from build123d import *

# Parameters (mm, degrees)
SKETCH1_W               = 984.25
SKETCH1_H               = 914.4
BOSS_EXTRUDE1_DEPTH     = 11.90625
CUT_EXTRUDE1_DEPTH      = 1
CUT_EXTRUDE1_DEPTH_BACK = 12.90625


with BuildPart() as part:
    # Sketch1 → Boss-Extrude1 (new body)
    with BuildSketch(Plane.XY):
        Rectangle(SKETCH1_W, SKETCH1_H)
    extrude(amount=BOSS_EXTRUDE1_DEPTH)

    # Sketch3 → Cut-Extrude1 (cut, two sides)
    with BuildSketch(Plane.XY.offset(11.90625)) as cut_extrude1_sk:
        Polygon((0, -406.4), (215.9, -406.4), (215.9, -215.9), (-215.9, -215.9), (-215.9, -406.4), align=None)
    extrude(amount=CUT_EXTRUDE1_DEPTH, mode=Mode.SUBTRACT)
    extrude(cut_extrude1_sk.sketch, amount=-CUT_EXTRUDE1_DEPTH_BACK, mode=Mode.SUBTRACT)


solid = part.part
Can you work these out from the model? Positions are in its coordinate system, mm. Coordinates: 2 decimals unless noted, no trailing zeros. Write each loop counter-clockwise with the first axis right and the second up, starting at its lowest first coordinate (ties: lowest second). Pieces come first, ordered by that corner, then holes.
Q1. Please list where these lines run through material, in increasing order: L1, parallel to Y at x = -163, z = 5.5; L2, parallel to X at y = -216.5, z = 10 (3 decimals).
Results found:
L1: y = -457.2 to -406.4, -215.9 to 457.2
L2: x = -492.125 to -215.9, 215.9 to 492.125
Q2. Imagine slicing it at C-C, the plane y = -371. List the corners of the cut face in (x, z) for me (3 decimals).
Results found:
outline: (-492.125, 0) - (-215.9, 0) - (-215.9, 11.906) - (-492.125, 11.906) - close; (215.9, 0) - (492.125, 0) - (492.125, 11.906) - (215.9, 11.906) - close
Q3. Imagine slicing it at B-B, the plane z = 6.25. List the corners of the cut face in (x, y) for me (3 decimals), plus the area to 3 significant figures.
Results found:
outline: (-492.125, -457.2) - (492.125, -457.2) - (492.125, 457.2) - (-492.125, 457.2) - close; hole (-215.9, -406.4) - (215.9, -406.4) - (215.9, -215.9) - (-215.9, -215.9) - close
area: 818,000 mm2
Q4. Imagine slicing it at A-A, the plane x = -136.5. List the corners of the cut face in (y, z) for me.
Results found:
outline: (-457.2, 0) - (-406.4, 0) - (-406.4, 11.91) - (-457.2, 11.91) - close; (-215.9, 0) - (457.2, 0) - (457.2, 11.91) - (-215.9, 11.91) - close
